from build123d import *

# Parameters (mm, degrees)
SKETCH1_R                = 12
BOSS_EXTRUDE1_DEPTH      = 73
SKETCH2_R                = 12
BOSS_EXTRUDE2_DEPTH      = 36.5
BOSS_EXTRUDE2_DEPTH_BACK = 36.5


with BuildPart() as part:
    # Sketch1 → Boss-Extrude1 (new body)
    with BuildSketch(Plane(origin=(0, 0, 0), x_dir=(1, 0, 0), z_dir=(0, 1, 0))):
        Circle(SKETCH1_R)
    extrude(amount=BOSS_EXTRUDE1_DEPTH)

    # Sketch2 → Boss-Extrude2 (add, two sides)
    with BuildSketch(Plane.XY) as boss_extrude2_sk:
        with Locations((0, 36.5)):
            Circle(SKETCH2_R)
    extrude(amount=BOSS_EXTRUDE2_DEPTH)
    extrude(boss_extrude2_sk.sketch, amount=-BOSS_EXTRUDE2_DEPTH_BACK)


solid = part.part
Could you check a few things on this model? Use its own coordinates, in mm. A direction names the side the tool comes from. Give positions to 0.01 mm unless a question says otherwise; leave off trailing zeros. Order: outer loops, then holes, each group sorted by start corner. A loop starts at its lowest first (then second) coordinate and runs counter-clockwise, first axis right, second up. Notation, with made-up numbers: (73.5, 84.5) - (99.5, 84.5) arc R31 cw to (99.5, 110.5) - close; hole circle Ø7 at (-28, 74). An arc over 180 degrees is marked (long way). One line per item, written item: value. Start each with the question number.
1. Imagine slicing it at D-D on x = -9.25. List the corners of the cut face in (y, z) for me, plus the area to 3 significant figures.
2. Imagine slicing it at B-B on y = 31. List the corners of the cut face in (x, z) for me.
3. Imagine slicing it at C-C on z = 4. List the corners of the cut face in (x, y) for me, plus the area to 3 significant figures.
4. If I drill on probe 1 along Y at (x, z) = (0, 26); probe 2 along X at (y, z) = (37, -13); probe 3 along Y at (x, z) = (3, 16.5), over which ranges is the centre line in solid material (lowest first)?
5. Imagine slicing it at A-A on x = 0. List the corners of the cut face in (y, z) for me.
6. For P1, Ø12, axis at x = 7.5, y = 63, coming from the -Z side; P2, Ø1.5, axis at y = 29, z = -1.5, coming from the -X side; P3, Ø8, axis at x = -2.5, z = -23, coming from the +Y side, each with a flat end and sliding along its axis, tell me the tip position at first contact or that it passes through.
7. For faces 1 (the face through (-11.99, 37.03, 22.05)), 2 (the face through (-1.56, 13.94, -11.9)), 3 (the face through (-11.99, 37.03, -22.05)), which set-ups out of +Z, -Z, +X, -X, +Y, -Y let a thin tool reach every point of the face, with its end or its side?
Values:
1. outline: (0, -7.64) - (28.86, -7.64) - (28.86, -36.5) - (44.14, -36.5) - (44.14, -7.64) - (73, -7.64) - (73, 7.64) - (44.14, 7.64) - (44.14, 36.5) - (28.86, 36.5) - (28.86, 7.64) - (0, 7.64) - close
1. area: 2,000 mm²
2. outline: (-10.67, -36.5) - (10.67, -36.5) - (10.67, -5.5) arc R12 ccw to (10.67, 5.5) - (10.67, 36.5) - (-10.67, 36.5) - (-10.67, 5.5) arc R12 ccw to (-10.67, -5.5) - close
3. outline: (-11.31, 0) - (11.31, 0) - (11.31, 32.5) arc R12 ccw to (11.31, 40.5) - (11.31, 73) - (-11.31, 73) - (-11.31, 40.5) arc R12 ccw to (-11.31, 32.5) - close
3. area: 1,660 mm²
4. probe 1: 24.5 to 48.5
4. probe 2: -11.99 to 11.99
4. probe 3: 24.88 to 48.12
5. outline: (0, -12) - (24.5, -12) - (24.5, -36.5) - (48.5, -36.5) - (48.5, -12) - (73, -12) - (73, 12) - (48.5, 12) - (48.5, 36.5) - (24.5, 36.5) - (24.5, 12) - (0, 12) - close
6. P1: z = -11.91
6. P2: x = -11.98
6. P3: y = 48.5
7. face 1: +Z
7. face 2: -Y
7. face 3: -Z
